Verification items for the finished model (mm, model axes). Face numbers are marked on the shaded views. A direction names the side the tool comes from. Round coordinates to 2 decimals unless told otherwise and drop trailing zeros. Order: outer loops, then holes, each group sorted by start corner. A loop starts at its lowest first (then second) coordinate and runs counter-clockwise, first axis right, second up. Notation, with made-up numbers: (-1, 56.5) -> (57, 56.5) arc R37 cw to (57, 92.5) -> close; hole circle Ø10 at (9.25, 85.25). An arc over 180 degrees is marked (long way). Put each result on its own line as item: value.
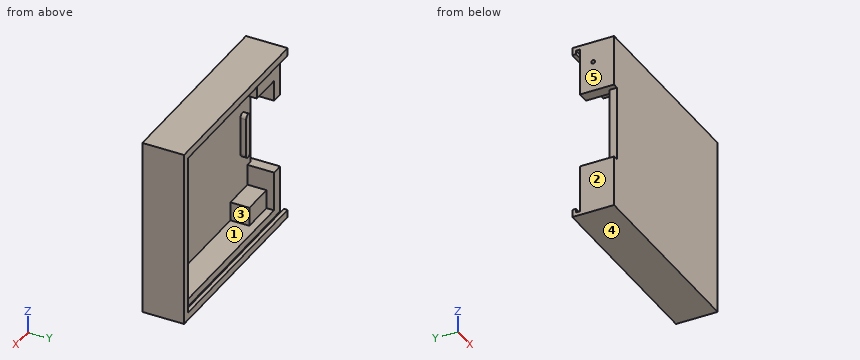
```python
from build123d import *

# Parameters (mm, degrees)
CROQUIS1_W               = 51.5
CROQUIS1_H               = 47
SALIENTE_EXTRUIR1_DEPTH  = 2
SALIENTE_EXTRUIR11_DEPTH = 1.5
CROQUIS3_W               = 51.5
CROQUIS3_H               = 47
CROQUIS3_W_2             = 45.5
CROQUIS3_H_2             = 41
SALIENTE_EXTRUIR10_DEPTH = 7
CROQUIS4_W               = 3
CROQUIS4_H               = 20
CORTAR_EXTRUIR3_DEPTH    = 7
CROQUIS5_W               = 8.5
CROQUIS5_H               = 5
SALIENTE_EXTRUIR12_DEPTH = 7
CROQUIS6_R               = 0.5
CORTAR_EXTRUIR2_DEPTH    = 12.5
CROQUIS8_W               = 8.5
CROQUIS8_H               = 5
SALIENTE_EXTRUIR13_DEPTH = 5
SALIENTE_EXTRUIR14_DEPTH = 2
CROQUIS10_W              = 50.5
CROQUIS10_H              = 1
SALIENTE_EXTRUIR15_DEPTH = 1
CROQUIS11_W              = 50.5
CROQUIS11_H              = 1
SALIENTE_EXTRUIR16_DEPTH = 1
CROQUIS12_W              = 43
CROQUIS12_H              = 1
SALIENTE_EXTRUIR17_DEPTH = 1
CROQUIS13_W              = 1.5
CROQUIS13_H              = 20
CORTAR_EXTRUIR4_DEPTH    = 3


with BuildPart() as part:
    # Croquis1 → Saliente-Extruir1 (new body)
    with BuildSketch(Plane(origin=(0, 0, 0), x_dir=(1, 0, 0), z_dir=(0, 1, 0))):
        with Locations((-25.75, 23.5)):
            Rectangle(CROQUIS1_W, CROQUIS1_H)
    extrude(amount=SALIENTE_EXTRUIR1_DEPTH)

    # Croquis2 → Saliente-Extruir11 (add)
    with BuildSketch(Plane(origin=(0, 2, 0), x_dir=(1, 0, 0), z_dir=(0, 1, 0))):
        with BuildLine():
            Line((-45, 28.5), (-45, 18.5))
            ThreePointArc((-45, 18.5), (-46, 17.5), (-47, 18.5))
            Line((-47, 18.5), (-47, 28.5))
            ThreePointArc((-47, 28.5), (-46, 29.5), (-45, 28.5))
        make_face()
    extrude(amount=SALIENTE_EXTRUIR11_DEPTH)

    # Croquis3 → Saliente-Extruir10 (add)
    with BuildSketch(Plane(origin=(0, 2, 0), x_dir=(1, 0, 0), z_dir=(0, 1, 0))):
        with Locations((-25.75, 23.5)):
            Rectangle(CROQUIS3_W, CROQUIS3_H)
        with Locations((-25.75, 23.5)):
            Rectangle(CROQUIS3_W_2, CROQUIS3_H_2, mode=Mode.SUBTRACT)
    extrude(amount=SALIENTE_EXTRUIR10_DEPTH)

    # Croquis4 → Cortar-Extruir3 (cut)
    with BuildSketch(Plane(origin=(0, 9, 0), x_dir=(1, 0, 0), z_dir=(0, 1, 0))):
        with Locations((-50, 23.5)):
            Rectangle(CROQUIS4_W, CROQUIS4_H)
    extrude(amount=-CORTAR_EXTRUIR3_DEPTH, mode=Mode.SUBTRACT)

    # Croquis5 → Saliente-Extruir12 (add)
    with BuildSketch(Plane(origin=(0, 2, 0), x_dir=(1, 0, 0), z_dir=(0, 1, 0))):
        with Locations((-44.25, 5.5)):
            Rectangle(CROQUIS5_W, CROQUIS5_H)
    extrude(amount=SALIENTE_EXTRUIR12_DEPTH)

    # Croquis6 → Cortar-Extruir2 (cut, through all)
    with BuildSketch(Plane(origin=(-40, 0, 0), x_dir=(0, 0, -1), z_dir=(1, 0, 0))):
        with Locations((5.5, 5.5)):
            Circle(CROQUIS6_R)
    extrude(amount=-CORTAR_EXTRUIR2_DEPTH, mode=Mode.SUBTRACT)

    # Croquis8 → Saliente-Extruir13 (add)
    with BuildSketch(Plane(origin=(0, 2, 0), x_dir=(1, 0, 0), z_dir=(0, 1, 0))):
        with Locations((-44.25, 41.5)):
            Rectangle(CROQUIS8_W, CROQUIS8_H)
    extrude(amount=SALIENTE_EXTRUIR13_DEPTH)

    # Croquis9 → Saliente-Extruir14 (add)
    with BuildSketch(Plane(origin=(0, 9, 0), x_dir=(1, 0, 0), z_dir=(0, 1, 0))):
        Polygon((-51.5, 1), (-1, 1), (-1, 46), (-51.5, 46), (-51.5, 47), (0, 47), (0, 0), (-51.5, 0), align=None)
    extrude(amount=SALIENTE_EXTRUIR14_DEPTH)

    # Croquis10 → Saliente-Extruir15 (add)
    with BuildSketch(Plane.XY.offset(-46)):
        with Locations((-26.25, 10.5)):
            Rectangle(CROQUIS10_W, CROQUIS10_H)
    extrude(amount=SALIENTE_EXTRUIR15_DEPTH)

    # Croquis11 → Saliente-Extruir16 (add)
    with BuildSketch(Plane(origin=(0, 0, -1), x_dir=(-1, 0, 0), z_dir=(0, 0, -1))):
        with Locations((26.25, 10.5)):
            Rectangle(CROQUIS11_W, CROQUIS11_H)
    extrude(amount=SALIENTE_EXTRUIR16_DEPTH)

    # Croquis12 → Saliente-Extruir17 (add)
    with BuildSketch(Plane.ZY.offset(1)):
        with Locations((-23.5, 10.5)):
            Rectangle(CROQUIS12_W, CROQUIS12_H)
    extrude(amount=SALIENTE_EXTRUIR17_DEPTH)

    # Croquis13 → Cortar-Extruir4 (cut, through all)
    with BuildSketch(Plane(origin=(0, 2, 0), x_dir=(1, 0, 0), z_dir=(0, 1, 0))):
        with Locations((-50.75, 23.5)):
            Rectangle(CROQUIS13_W, CROQUIS13_H)
    extrude(amount=-CORTAR_EXTRUIR4_DEPTH, mode=Mode.SUBTRACT)


solid = part.part
```
Item 1: Sectioned sample at A-A, the plane z = -15.5. Record the boundary of the cut face in (x, y), then the cut area to 3 significant figures.
Geometry check:
outline: (-50, 0) -> (0, 0) -> (0, 11) -> (-2, 11) -> (-2, 10) -> (-1, 10) -> (-1, 9) -> (-3, 9) -> (-3, 2) -> (-50, 2) -> close
area: 124 mm2
Item 2: Sectioned sample at D-D, the plane z = -41.5. Record the boundary of the cut face in (x, y), then the cut area to 4 significant figures.
Geometry check:
outline: (-51.5, 0) -> (0, 0) -> (0, 11) -> (-2, 11) -> (-2, 10) -> (-1, 10) -> (-1, 9) -> (-3, 9) -> (-3, 2) -> (-40, 2) -> (-40, 7) -> (-48.5, 7) -> (-48.5, 9) -> (-51.5, 9) -> close
area: 190.5 mm2
Item 3: Tool access check on the marked faces 1 and 2. Record the directions out of +Z, -Z, +X, -X, +Y, -Y that give a thin tool (end or side, any length) a straight path to the whole face; none if there is none.
Geometry check:
face 1: +Y
face 2: +Z, -Z, -X, +Y, -Y
Item 4: Depth check by flat-ended pin: pin 1 Ø3 at (x, y) = (-39, 5) entering from +Z; pin 2 Ø3 at (y, z) = (7, -31.5) entering from -X; pin 3 Ø3.5 at (y, z) = (4.5, -30) entering from -X; pin 4 Ø6 at (y, z) = (1, -23) entering from -X. Enter the tip coordinate at first touch or a pass-through.
Geometry check:
pin 1: z = 0
pin 2: x = -3
pin 3: x = -47
pin 4: x = -50
Item 5: Sectioned sample at C-C, the plane z = -25.5. Record the boundary of the cut face in (x, y), then the cut area to 3 significant figures.
Geometry check:
outline: (-50, 0) -> (0, 0) -> (0, 11) -> (-2, 11) -> (-2, 10) -> (-1, 10) -> (-1, 9) -> (-3, 9) -> (-3, 2) -> (-45, 2) -> (-45, 3.5) -> (-47, 3.5) -> (-47, 2) -> (-50, 2) -> close
area: 127 mm2
Item 6: Release check for a two-part mould opening along X. For the marked faces 3, 4 and 5 record: pulls with the +X half, pulls with the -X half, needs draft (parallel to the pull), parting line crosses it, or undercut.
Geometry check:
face 3: undercut
face 4: needs draft
face 5: pulls with the -X half
Item 7: Sectioned sample at B-B, the plane x = -6.5. Record the boundary of the cut face in (y, z).
Geometry check:
outline: (0, -47) -> (11, -47) -> (11, -45) -> (10, -45) -> (10, -46) -> (9, -46) -> (9, -44) -> (2, -44) -> (2, -3) -> (9, -3) -> (9, -1) -> (10, -1) -> (10, -2) -> (11, -2) -> (11, 0) -> (0, 0) -> close
Item 8: Material ranges on line 1 along Y through (x, z) = (-47.75, -5.5); line 2 along Z through (x, y) = (-37.5, 2.5); line 3 along X through (y, z) = (5, -10), recorded low to high.
Geometry check:
line 1: 0 to 5, 6 to 9
line 2: -47 to -44, -3 to 0
line 3: -51.5 to -48.5, -3 to 0
